Design review of the part built by this model. Coordinates are the model's own, in mm. Give positions to 0.01 mm unless a question says otherwise; leave off trailing zeros. Loops run counter-clockwise (first coordinate to the right, second up) from the corner with the lowest first, then second, coordinate; pieces in that order, holes last. Notation, with made-up numbers: (17, -6.5) - (35, -6.5) arc R22 cw to (35, 31.5) - close; hole circle Ø3 at (34.5, 73.25). An arc over 180 degrees is marked (long way). Write each question's results on one line, items separated by ' | '.
from build123d import *

# Parameters (mm, degrees)
SKETCH1_W               = 635
SKETCH1_H               = 101.6
BOSS_EXTRUDE1_DEPTH     = 25.908
CUT_EXTRUDE1_START      = -26.908
SKETCH1_3_R             = 9.525
CUT_EXTRUDE1_DEPTH      = 27.908
LPATTERN1_COUNT         = 15
LPATTERN1_PITCH         = 40.386
SKETCH2_R               = 9.525
CUT_EXTRUDE2_DEPTH      = 1
CUT_EXTRUDE2_DEPTH_BACK = 26.908


with BuildPart() as part:
    # Sketch1 → Boss-Extrude1 (new body)
    with BuildSketch(Plane(origin=(0, 0, 0), x_dir=(1, 0, 0), z_dir=(0, 1, 0))):
        with Locations((-281.432, 0.0508)):
            Rectangle(SKETCH1_W, SKETCH1_H)
    extrude(amount=-BOSS_EXTRUDE1_DEPTH)

    # Sketch1<3> → Cut-Extrude1 (cut)
    with BuildSketch(Plane(origin=(0, 0, 0), x_dir=(1, 0, 0), z_dir=(0, 1, 0)).offset(CUT_EXTRUDE1_START)):
        Circle(SKETCH1_3_R)
        with Locations((20.193, 34.9758)):
            Circle(SKETCH1_3_R)
        with Locations((20.193, -34.9758)):
            Circle(SKETCH1_3_R)
    cut_extrude1 = extrude(amount=CUT_EXTRUDE1_DEPTH, mode=Mode.SUBTRACT)

    # LPattern1: Cut-Extrude1 ×15
    with Locations(*[(-i * LPATTERN1_PITCH, 0, 0) for i in range(1, LPATTERN1_COUNT)]):
        add(cut_extrude1, mode=Mode.SUBTRACT)

    # Sketch2 → Cut-Extrude2 (cut, two sides)
    with BuildSketch(Plane(origin=(0, 0, 0), x_dir=(1, 0, 0), z_dir=(0, 1, 0))) as cut_extrude2_sk:
        with Locations((-585.597, 34.9758)):
            Circle(SKETCH2_R)
        with Locations((-585.597, -34.9758)):
            Circle(SKETCH2_R)
    extrude(amount=CUT_EXTRUDE2_DEPTH, mode=Mode.SUBTRACT)
    extrude(cut_extrude2_sk.sketch, amount=-CUT_EXTRUDE2_DEPTH_BACK, mode=Mode.SUBTRACT)


solid = part.part
(1) Wall thickness on line 1 along Z through (x, y) = (-262, -9.75); line 2 along Z through (x, y) = (-544, -2.25); line 3 along Z through (x, y) = (-83.5, -3): over which ranges is each line inside the solid? List them lowest first. Write a range as from..to.
Answers below:
line 1: -50.85..-44.49, -25.46..25.46, 44.49..50.75 | line 2: -50.85..-44.42, -25.53..25.53, 44.42..50.75 | line 3: -50.85..-9.13, 9.13..50.75
(2) Draft analysis for pull direction X (two halves, no side actions). For faces 1 (the flat face through (-286, -13, 50.749)), 2 (the cylindrical face through (-21.43, -13.14, 25.53)), state which applies: pulls with the +X half, pulls with the -X half, needs draft (parallel to the pull), parting line crosses it, or undercut.
Answers below:
face 1: needs draft | face 2: undercut
(3) Take a section at B-B on z = 0. Count the separate pieces of the cut face and the enclosed holes in it, plus the area to 3 significant figures.
Answers below:
separate pieces: 16 | enclosed holes: 0 | area: 9,050 mm2
(4) Insertion check: P1, Ø8, axis at x = -155.5, z = 2, coming from the +Y side. The pin has a flat end and moves straight along its axis. Give the tip position at first contact, or say it passes through.
Answers below:
P1: y = 0
(5) Take a section at C-C on x = -201.5. Give the boundary of the cut face in (y, z).
Answers below:
outline: (-25.91, -50.85) - (0, -50.85) - (0, -9.52) - (-25.91, -9.52) - close; (-25.91, 9.52) - (0, 9.52) - (0, 50.75) - (-25.91, 50.75) - close
(6) Take a section at A-A on x = -403.86. Give the boundary of the cut face in (y, z) (3 decimals).
Answers below:
outline: (-25.908, -50.851) - (0, -50.851) - (0, -9.525) - (-25.908, -9.525) - close; (-25.908, 9.525) - (0, 9.525) - (0, 50.749) - (-25.908, 50.749) - close
